Input: dimensioned drawing with shaded views. Units: mm. Origin: part minimum x, y, z. Round coordinates to 2 decimals unless told otherwise and drop trailing zeros. Order: outer loops, then holes, each group sorted by start corner. A loop starts at its lowest first (then second) coordinate and runs counter-clockwise, first axis right, second up. Notation, with made-up numbers: M 31.5,30.25 L 67.5,30.25 A22 cw 67.5,62.25 Z; hole C -27,42.5 d9. An arc over 180 degrees is marked long. Put each result on its own line as item: value. Start each with the question number.
1) Section A-A, the plane y = 3. Return loops of the section in (x, z).
2) Material intervals for probe 1 along Y at (x, z) = (9, 0.5); probe 2 along X at (y, z) = (3, 0.75), sorted ascending. Write a range as [from, to].
3) Section B-B, the plane x = 9. Return loops of the section in (y, z).
4) First-contact query: P1, Ø2.5, axis at x = 54, y = 45, coming from the -Z side. Flat tip, straight axial feed; report the tip coordinate or a pass-through.
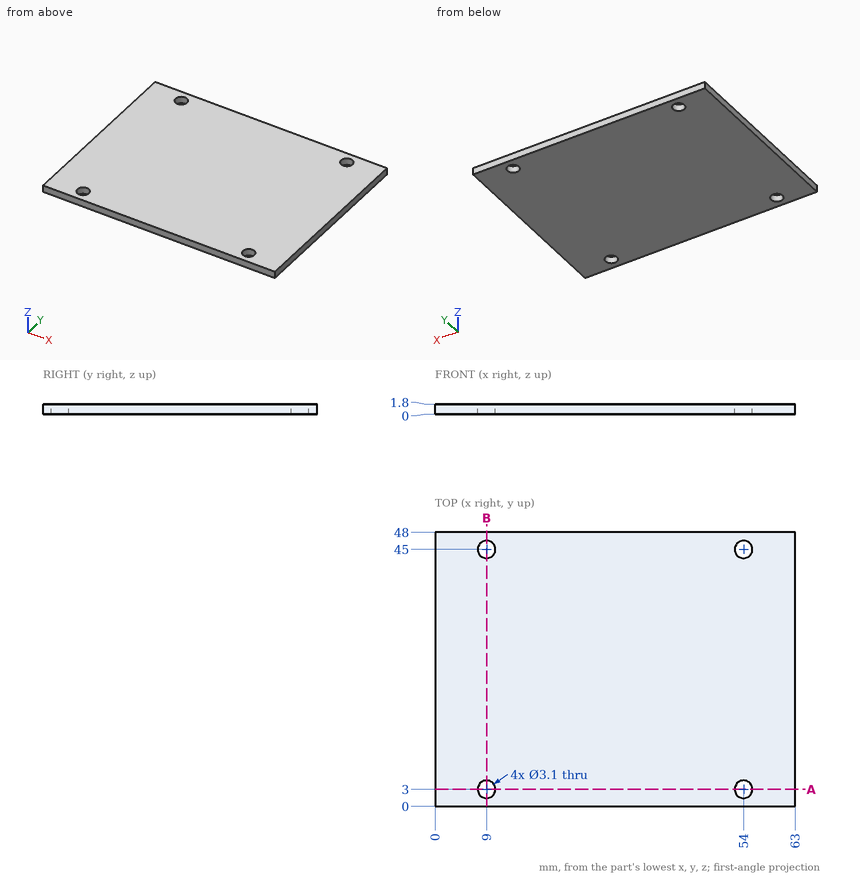
Result sheet:
1. outline: M 0,0 L 7.45,0 L 7.45,1.8 L 0,1.8 Z; M 10.55,0 L 52.45,0 L 52.45,1.8 L 10.55,1.8 Z; M 55.55,0 L 63,0 L 63,1.8 L 55.55,1.8 Z
2. probe 1: y = [0, 1.45], [4.55, 43.45], [46.55, 48]
2. probe 2: x = [0, 7.45], [10.55, 52.45], [55.55, 63]
3. outline: M 0,0 L 1.45,0 L 1.45,1.8 L 0,1.8 Z; M 4.55,0 L 43.45,0 L 43.45,1.8 L 4.55,1.8 Z; M 46.55,0 L 48,0 L 48,1.8 L 46.55,1.8 Z
4. P1: passes through
